Autodesk Inventor part; units mm, degrees
ref_plane "YZ Plane" through (0, 0, 0) normal (1, 0, 0) x (0, 1, 0)
ref_plane "XZ Plane" through (0, 0, 0) normal (0, 1, 0) x (-1, 0, 0)
ref_plane "XY Plane" through (0, 0, 0) normal (0, 0, 1) x (1, 0, 0)
sketch "Sketch1" plane through (0, 0, 0) normal (0, 1, 0) x (-1, 0, 0)
  circle A0 centre (0, 0) radius 420
  circle A1 centre (0, 0) radius 360
  circle A2 centre (390, 0) radius 7.1437
  circle A3 centre (0, 0) radius 390 construction
  dimension "d3" = 780
  dimension "d0" = 840
  dimension "d1" = 720
  dimension "d2" = 14.2875
extrude "Extrusion1" add sketch "Sketch1" along normal blind 8 contours A0 | A2
hole "Hole1" at (-390, 0, 0) direction (0, 1, 0) diameter 14.2875 end through all
pattern_circular "Circular Pattern1" count 24 over 360 about axis through (0, 0, 0) along (0, 1, 0) of "Hole1"
equation "\"d6\" = d2"
properties part number "Tapa1" material "Steel ASTM A36"
Here's how the part is built. I have some questions about the finished solid (model axes, mm). Coordinates: 2 decimals unless noted, no trailing zeros. Write each loop counter-clockwise with the first axis right and the second up, starting at its lowest first coordinate (ties: lowest second). Pieces come first, ordered by that corner, then holes.
Item 1: I want a section at A-A on x = 171. Write out the boundary of the cut face in (y, z).
Item 2: Will these pins go through, and if not, where does the flat tip stop? pin 1 (4 mm diameter, centred on y = 7, z = -304, fed in from -X); pin 2 (1.5 mm diameter, centred on x = -60, y = 5.5, fed in from +Z); pin 3 (1.5 mm diameter, centred on y = 7, z = -273.5, fed in from -X).
Item 3: If I drill on line 1 (Z direction, x = 0, y = 2.75); line 2 (X direction, y = 0.5, z = -196); line 3 (Z direction, x = 102.5, y = 6.25), over which ranges is the centre line in solid material (lowest first)?
Item 4: I want a section at B-B on z = 22. Write out the boundary of the cut face in (x, y), and give its area (3 significant figures).
Item 5: If we mould it in two halves opening along Z, with no side actions, what happens to faces 1 (the cylindrical face through (-400.605, 3.944, -126.157)), 2 (the cylindrical face through (-166.12, 3.94, 319.38)), 3 (the flat face through (-309.2, 8, -184.7))? For each: +Z half, -Z half, draft (parallel to the pull), parting line (faces both ways), or undercut.
Item 6: I want a section at C-C on y = 6.5. Count the separate pieces of the cut face and the enclosed holes in it, and give its area (3 significant figures).
Findings below:
1. outline: (0, -383.61) - (8, -383.61) - (8, -316.79) - (0, -316.79) - close; (0, 316.79) - (8, 316.79) - (8, 383.61) - (0, 383.61) - close
2. pin 1: stops at x = -291.88
2. pin 2: stops at z = 415.8
2. pin 3: stops at x = -319.39
3. line 1: z = -420 to -397.14, -382.86 to -360, 360 to 382.86, 397.14 to 420
3. line 2: x = -371.46 to -344.82, -330.68 to -301.97, 301.97 to 330.68, 344.82 to 371.46
3. line 3: z = -407.3 to -383.68, -369.74 to -345.1, 345.1 to 369.74, 383.68 to 407.3
4. outline: (-419.42, 0) - (-359.33, 0) - (-359.33, 8) - (-419.42, 8) - close; (359.33, 0) - (419.42, 0) - (419.42, 8) - (359.33, 8) - close
4. area: 962 mm2
5. face 1: parting line
5. face 2: undercut
5. face 3: draft
6. separate pieces: 1
6. enclosed holes: 25
6. area: 143,000 mm2
